Here's the drawing with two shaded views (mm, measured from the low corner). I have some questions. Coordinates: 2 decimals unless noted, no trailing zeros. Loops run counter-clockwise (first coordinate to the right, second up) from the corner with the lowest first, then second, coordinate; pieces in that order, holes last. Notation, with made-up numbers: M 53,-5.75 L 84,-5.75 A24 cw 84,28.25 Z; hole C -22,74 d1. An arc over 180 degrees is marked long. Use one line per item in the form item = value. Start each with the question number.
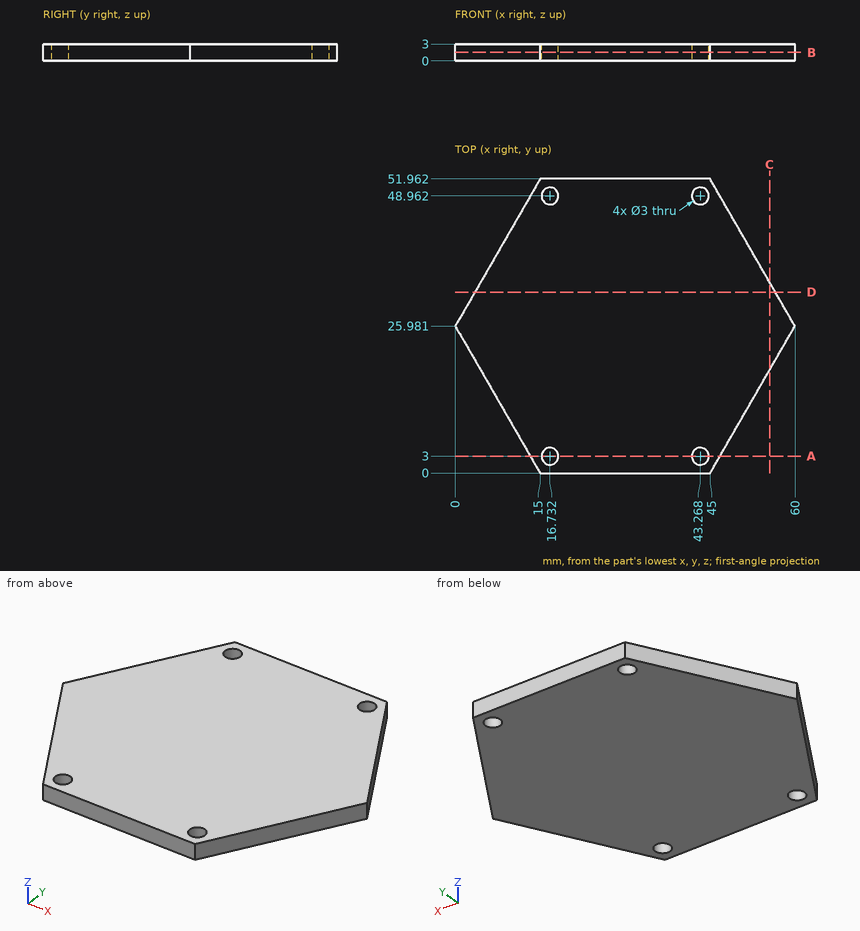
Item 1: I'm going to push flat-ended pins straight in: P1, Ø1.5, axis at y = 20, z = 2.5, coming from the -X side; P2, Ø2.5, axis at x = 16.73, y = 3, coming from the +Z side; P3, Ø1, axis at y = 44, z = 1, coming from the +X side (1 decimal). Where does each tip first touch, or does it pass through?
Item 2: I want a section at A-A (y = 3). Write out the boundary of the cut face in (x, z).
Item 3: I want a section at B-B (z = 1.5). Write out the boundary of the cut face in (x, y).
Item 4: Please list where these lines run through material, in increasing order: line 1 along X through (y, z) = (48.5, 1.65) (1 decimal); line 2 along Y through (x, z) = (16, 0.4); line 3 along X through (y, z) = (26, 0.85).
Item 5: I want a section at C-C (x = 55.5). Write out the boundary of the cut face in (y, z) (1 decimal).
Item 6: I want a section at D-D (y = 32). Write out the boundary of the cut face in (x, z) (1 decimal), plus the area to 3 significant figures.
Worked answers:
q1.P1 = 3.02
q1.P2 = through
q1.P3 = 49.9
q2.outline = M 13.27,0 L 15.23,0 L 15.23,3 L 13.27,3 Z; M 18.23,0 L 41.77,0 L 41.77,3 L 18.23,3 Z; M 44.77,0 L 46.73,0 L 46.73,3 L 44.77,3 Z
q3.outline = M 0,25.98 L 15,0 L 45,0 L 60,25.98 L 45,51.96 L 15,51.96 Z; hole C 16.73,3 d3; hole C 16.73,48.96 d3; hole C 43.27,3 d3; hole C 43.27,48.96 d3
q4.line_1 = 13 to 15.3, 18.2 to 41.8, 44.7 to 47
q4.line_2 = 0 to 1.69, 4.31 to 47.65, 50.27 to 51.96
q4.line_3 = 0.01 to 59.99
q5.outline = M 18.2,0 L 33.8,0 L 33.8,3 L 18.2,3 Z
q6.outline = M 3.5,0 L 56.5,0 L 56.5,3 L 3.5,3 Z
q6.area = 159 mm²
